Check sheet for the modelled part. Datum: model origin and axes. Units: mm. A direction names the side the tool comes from. Give positions to 0.01 mm unless a question says otherwise; leave off trailing zeros. Order: outer loops, then holes, each group sorted by start corner. A loop starts at its lowest first (then second) coordinate and runs counter-clockwise, first axis right, second up.
Item 1: Sectioned sample at B-B on y = -29.5. Record the boundary of the cut face in (x, z).
Item 2: Material ranges on line 1 along Z through (x, y) = (2.25, -6); line 2 along Z through (x, y) = (-3.25, 1.5); line 3 along Z through (x, y) = (4.75, -28.5), recorded low to high.
Item 3: Release check for a two-part mould opening along Y. For faces 1 (the flat face through (-6, -20, 0)), 2 (the flat face through (3, 0, -4.144)), 3 (the flat face through (0, 20, 11)) record: released by +Y, released by -Y, zero draft, split by the parting line, or undercut.
Item 4: Gauge pin test, flat ends, axial feed: P1, Ø2.5, axis at x = 0, y = -32.5, coming from the -Z side; P2, Ø6.5, axis at x = -5.5, z = 2.5, coming from the -Y side; P3, Ø1.8, axis at x = -4, z = -3.5, coming from the +Y side. Record the tip position at first contact, or that the pin passes through.
Item 5: Sectioned sample at A-A on y = -8. Record the boundary of the cut face in (x, z), and give its area (3 significant figures).
Item 6: Access from +Z, -Z, +X, -X, +Y, -Y to the whole of each face (thin tool, end or side, straight path). Record for faces 4 (the flat face through (6, 20, 0)), 5 (the flat face through (0, -20, 11)), 6 (the flat face through (3.5, 0, 0)).
Item 7: Sectioned sample at C-C on x = -2.75. Count the separate pieces of the cut face and the enclosed holes in it, and give its area (3 significant figures).
from build123d import *

# Parameters (mm, degrees)
BOSS_EXTRUDE1_START  = -20
SKETCH1_W            = 15
SKETCH1_H            = 30
SKETCH1_W_2          = 2
SKETCH1_H_2          = 4.496327887
SKETCH1_H_3          = 4
BOSS_EXTRUDE1_DEPTH  = 40
SKETCH2_W            = 15
SKETCH2_H            = 6
BOSS_EXTRUDE2_DEPTH  = 20
FILLET1_R            = 7.5
SKETCH3_R            = 1.5
CUT_EXTRUDE1_DEPTH   = 51.55937104
FILLET1_OF_MIRROR1_R = 7.5
FILLET4_R            = 3


with BuildPart() as part:
    # Sketch1 → Boss-Extrude1 (new body)
    with BuildSketch(Plane(origin=(0, 0, 0), x_dir=(1, 0, 0), z_dir=(0, 1, 0)).offset(BOSS_EXTRUDE1_START)):
        Rectangle(SKETCH1_W, SKETCH1_H)
        Polygon((-5.5, -13), (5.5, -13), (5.5, -4), (1.5, -4), (1.5, 4.144450542), (5.5, 4.144450542), (5.5, 13), (-5.5, 13), (-5.5, 4.144450542), (-1.5, 4.144450542), (-1.5, -4.208461458), (-5.5, -4.208461458), align=None, mode=Mode.SUBTRACT)
        with Locations((-4.5, -0.248163944)):
            Rectangle(SKETCH1_W_2, SKETCH1_H_2, mode=Mode.SUBTRACT)
        with Locations((4.5, 0)):
            Rectangle(SKETCH1_W_2, SKETCH1_H_3, mode=Mode.SUBTRACT)
    extrude(amount=BOSS_EXTRUDE1_DEPTH)

    # Sketch2 → Boss-Extrude2 (add)
    with BuildSketch(Plane.XZ.offset(20)):
        with Locations((0, 12)):
            Rectangle(SKETCH2_W, SKETCH2_H)
        with Locations((0, -12)):
            Rectangle(SKETCH2_W, SKETCH2_H)
    boss_extrude2 = extrude(amount=BOSS_EXTRUDE2_DEPTH)

    # Fillet1
    fillet1_edges = [part.edges().sort_by_distance(p)[0] for p in [
        (-7.5, -40, 12),
        (-7.5, -40, -12),
        (7.5, -40, -12),
        (7.5, -40, 12),
    ]]
    fillet(fillet1_edges, radius=FILLET1_R - 0.0001)  # a hair under: the kernel refuses the full size

    # Sketch3 → Cut-Extrude1 (cut, through all)
    with BuildSketch(Plane.XY.offset(15)):
        with Locations((0, -32.5)):
            Circle(SKETCH3_R)
    cut_extrude1 = extrude(amount=-CUT_EXTRUDE1_DEPTH, mode=Mode.SUBTRACT)

    # Mirror1: Boss-Extrude2, Cut-Extrude1 across plane
    add(boss_extrude2.mirror(Plane.ZX))
    add(cut_extrude1.mirror(Plane.ZX), mode=Mode.SUBTRACT)

    # Fillet1 of Mirror1
    fillet1_of_mirror1_edges = [part.edges().sort_by_distance(p)[0] for p in [
        (-7.5, 40, 12),
        (-7.5, 40, -12),
        (7.5, 40, -12),
        (7.5, 40, 12),
    ]]
    fillet(fillet1_of_mirror1_edges, radius=FILLET1_OF_MIRROR1_R - 0.0001)  # a hair under: the kernel refuses the full size

    # Fillet4
    fillet4_edges = [part.edges().sort_by_distance(p)[0] for p in [
        (5.303330148, -37.803330148, 15),
        (-5.303330148, -37.803330148, 15),
        (5.303330148, -37.803330148, -15),
        (-5.303330148, -37.803330148, -15),
        (-7.5, 0, 15),
        (-7.5, 0, -15),
        (7.5, 0, 15),
        (5.303330148, 37.803330148, 15),
        (-5.303330148, 37.803330148, 15),
        (7.5, 0, -15),
        (5.303330148, 37.803330148, -15),
        (-5.303330148, 37.803330148, -15),
    ]]
    fillet(fillet4_edges, radius=FILLET4_R)


solid = part.part
Report:
1. outline: (-7.5, -12) arc R3 ccw to (-4.5, -15) - (4.5, -15) arc R3 ccw to (7.5, -12) - (7.5, -9) - (-7.5, -9) - close; (-7.5, 9) - (7.5, 9) - (7.5, 12) arc R3 ccw to (4.5, 15) - (-4.5, 15) arc R3 ccw to (-7.5, 12) - close
2. line 1: z = -15 to -13, -4.14 to 4, 13 to 15
2. line 2: z = -15 to -13, -4.14 to 4.21, 13 to 15
2. line 3: z = -14.99 to -9, 9 to 14.99
3. face 1: released by -Y
3. face 2: zero draft
3. face 3: undercut
4. P1: passes through
4. P2: stops at y = -20
4. P3: stops at y = 20
5. outline: (-7.5, -12) arc R3 ccw to (-4.5, -15) - (4.5, -15) arc R3 ccw to (7.5, -12) - (7.5, 12) arc R3 ccw to (4.5, 15) - (-4.5, 15) arc R3 ccw to (-7.5, 12) - close; hole (-5.5, -13) - (5.5, -13) - (5.5, -4.14) - (1.5, -4.14) - (1.5, 4) - (5.5, 4) - (5.5, 13) - (-5.5, 13) - (-5.5, 4.21) - (-1.5, 4.21) - (-1.5, -4.14) - (-5.5, -4.14) - close; hole (-5.5, -2) - (-3.5, -2) - (-3.5, 2.5) - (-5.5, 2.5) - close; hole (3.5, -2) - (5.5, -2) - (5.5, 2) - (3.5, 2) - close
5. area: 205 mm2
6. face 4: +X, -X, +Y
6. face 5: none
6. face 6: +Y, -Y
7. separate pieces: 3
7. enclosed holes: 0
7. area: 953 mm2
